Part model, mm, in its own coordinate system. Round coordinates to 2 decimals unless told otherwise and drop trailing zeros. Order: outer loops, then holes, each group sorted by start corner. A loop starts at its lowest first (then second) coordinate and runs counter-clockwise, first axis right, second up. Notation, with made-up numbers: (82.5, -24.75) - (104.5, -24.75) arc R29 ccw to (104.5, 1.25) - close; hole circle Ø9 at (25.25, 41.25). An arc over 180 degrees is marked (long way). Answer as a JSON object with one key per item and string values.
Autodesk Inventor part; units mm, degrees
ref_plane "YZ Plane" through (0, 0, 0) normal (1, 0, 0) x (0, 1, 0)
ref_plane "XZ Plane" through (0, 0, 0) normal (0, 1, 0) x (-1, 0, 0)
ref_plane "XY Plane" through (0, 0, 0) normal (0, 0, 1) x (1, 0, 0)
sketch "Sketch1" plane through (0, 0, 0) normal (0, 1, 0) x (-1, 0, 0)
  line L0 (0, 0) -> (28.63, 0)
  line L1 (28.63, 0) -> (28.63, -41.25) construction
  line L2 (28.63, -41.25) -> (0, -41.25)
  line L3 (0, -41.25) -> (0, 0)
  line L4 (28.63, 6.675) -> (31.43, 6.675)
  line L5 (31.43, 6.675) -> (31.43, 0)
  line L6 (31.43, -47.925) -> (28.63, -47.925)
  line L7 (28.63, -47.925) -> (28.63, -41.25)
  line L8 (31.43, -20.625) -> (28.63, -20.625) construction
  line L9 (38.98, 0) -> (31.43, 0)
  line L10 (31.43, 0) -> (31.43, -41.25) construction
  line L11 (31.43, -41.25) -> (35.18, -41.25)
  line L12 (38.98, -41.25) -> (38.98, -34.5) construction
  line L13 (31.43, -41.25) -> (35.18, -41.25) construction
  line L14 (38.98, 0) -> (38.98, -1) construction
  line L15 (38.98, -34.5) -> (35.18, -41.25)
  line L16 (38.98, -34.5) -> (38.98, -33)
  line L17 (35.18, -41.25) -> (38.98, -41.25) construction
  line L18 (38.98, 0) -> (38.98, -1) construction
  line L19 (38.98, -1) -> (39.98, -1)
  line L20 (39.98, -1) -> (39.98, -4)
  line L21 (39.98, -33) -> (38.98, -33)
  line L22 (38.98, -33) -> (38.98, -1) construction
  line L23 (38.98, -1) -> (38.98, -33) construction
  line L24 (38.98, -33) -> (38.98, -34.5) construction
  line L25 (38.98, -1) -> (38.98, 0)
  line L26 (38.98, -33) -> (38.98, -1) construction
  line L27 (31.43, 0) -> (31.43, -41.25) construction
  line L28 (31.43, -41.25) -> (31.43, -47.925)
  line L29 (28.63, -41.25) -> (28.63, 0) construction
  line L30 (28.63, 0) -> (28.63, 6.675)
  line L31 (28.63, 0) -> (31.43, 0) construction
  line L32 (31.43, -41.25) -> (28.63, -41.25) construction
  line L33 (39.98, -1) -> (39.98, -4) construction
  line L34 (39.98, -4) -> (41.28, -4)
  line L35 (41.28, -4) -> (41.28, -16.6)
  line L36 (41.28, -16.6) -> (39.98, -16.6)
  line L37 (39.98, -16.6) -> (39.98, -4) construction
  line L38 (39.98, -4) -> (39.98, -16.6) construction
  line L39 (39.98, -16.6) -> (39.98, -33)
  line L40 (41.68, -17) -> (41.68, -3.6)
  line L41 (41.68, -3.6) -> (40.38, -3.6)
  line L42 (40.38, -3.6) -> (40.38, -0.6)
  line L43 (40.38, -0.6) -> (39.38, -0.6)
  line L44 (39.38, -0.6) -> (39.38, 0.4)
  line L45 (39.38, 0.4) -> (31.83, 0.4)
  line L46 (31.83, 0.4) -> (31.83, 7.075)
  line L47 (31.83, 7.075) -> (28.23, 7.075)
  line L48 (28.23, 7.075) -> (28.23, 0.4)
  line L49 (28.23, 0.4) -> (-0.4, 0.4)
  line L50 (-0.4, 0.4) -> (-0.4, -41.65)
  line L51 (-0.4, -41.65) -> (28.23, -41.65)
  line L52 (28.23, -41.65) -> (28.23, -48.325)
  line L53 (28.23, -48.325) -> (31.83, -48.325)
  line L54 (31.83, -48.325) -> (31.83, -41.65)
  line L55 (31.83, -41.65) -> (35.4138, -41.65)
  line L56 (35.4138, -41.65) -> (39.38, -34.6049)
  line L57 (39.38, -34.6049) -> (39.38, -33.4)
  line L58 (39.38, -33.4) -> (40.38, -33.4)
  line L59 (40.38, -33.4) -> (40.38, -17)
  line L60 (40.38, -17) -> (41.68, -17)
  line L61 (0, -20.625) -> (39.98, -20.625) construction
  line L62 (44.99, 9.375) -> (-5.01, 9.375)
  line L63 (-5.01, 9.375) -> (-5.01, -50.625)
  line L64 (-5.01, -50.625) -> (44.99, -50.625)
  line L65 (44.99, -50.625) -> (44.99, 9.375)
  line L66 (19.99, 9.375) -> (19.99, -50.625) construction
  point P0 (30.03, 6.675)
  point P1 (19.99, -20.625)
  dimension "d0" = 28.63
  dimension "d1" = 41.25
  dimension "d2" = 2.8
  dimension "d3" = 54.6
  dimension "d4" = 7.55
  dimension "d5" = 41.25
  dimension "d6" = 3.75
  dimension "d7" = 34.5
  dimension "d8" = 1
  dimension "d9" = 32
  dimension "d10" = 1
  dimension "d11" = 6.675
  dimension "d12" = 3
  dimension "d13" = 1.3
  dimension "d14" = 12.6
  dimension "d15" = 0.4
  dimension "d16" = 50
  dimension "d17" = 60
extrude "Extrusion1" add sketch "Sketch1" along normal blind 5 contours L65 L64 L63 L62
sketch "Sketch2" plane through (0, 5, 0) normal (0, 1, 0) x (1, 0, 0)
  line L0 (-44.99, 50.625) -> (-44.99, -9.375)
  line L1 (5.01, 50.625) -> (-44.99, 50.625)
  line L2 (-44.99, -9.375) -> (-41.68, -9.375)
  line L3 (-41.68, -9.375) -> (-41.68, 50.625)
  line L4 (-41.68, 50.625) -> (-44.99, 50.625)
  line L5 (-44.99, 50.625) -> (-44.99, -9.375)
  point P0 (0, 0)
  dimension "d20" = 3.31
extrude "Extrusion2" cut sketch "Sketch2" against normal through all
sketch "Sketch3" plane through (0, 0, 0) normal (0, -1, 0) x (1, 0, 0)
  line L0 (5.01, 9.375) -> (5.01, -50.625)
  line L1 (-41.68, -17) -> (-41.68, -50.625)
  line L2 (5.01, 9.375) -> (-41.68, 9.375)
  line L3 (-41.68, 9.375) -> (-41.68, -50.625)
  line L4 (-41.68, -50.625) -> (5.01, -50.625)
  line L5 (5.01, -50.625) -> (5.01, 9.375)
  point P0 (0, 0)
extrude "Extrusion3" add sketch "Sketch3" along normal blind 4
sketch "Sketch4" plane through (-41.68, 5, 9.375) normal (0, 0, 1) x (1, 0, 0)
  line L0 (0, 0) -> (0, -9)
  line L1 (46.69, -9) -> (46.69, 0)
  line L2 (0, 0) -> (46.69, 0)
  line L3 (46.69, 0) -> (46.69, -9)
  line L4 (46.69, -9) -> (0, -9)
  line L5 (0, -9) -> (0, 0)
  point P0 (41.68, -5)
extrude "Extrusion4" add sketch "Sketch4" along normal blind 10
sketch "Sketch5" plane through (5.01, 5, -50.625) normal (0, 0, -1) x (-1, 0, 0)
  line L0 (0, 0) -> (46.69, 0)
  line L1 (46.69, 0) -> (46.69, -9)
  line L2 (0, 0) -> (46.69, 0)
  line L3 (46.69, 0) -> (46.69, -9)
  line L4 (46.69, -9) -> (0, -9)
  line L5 (0, -9) -> (0, 0)
  point P0 (5.01, -5)
extrude "Extrusion5" add sketch "Sketch5" along normal blind 10
sketch "Sketch6" plane through (0, -4, 0) normal (0, -1, 0) x (1, 0, 0)
  line L0 (-41.68, 19.375) -> (5.01, 19.375)
  line L1 (5.01, 19.375) -> (0.01, 19.375)
  line L2 (0.01, 14.375) -> (0.01, 10.375)
  line L3 (0.01, 10.375) -> (5.01, 10.375)
  line L4 (5.01, 10.375) -> (5.01, 19.375)
  line L5 (5.01, 19.375) -> (-3.99, 19.375)
  line L6 (-3.99, 19.375) -> (-3.99, 14.375)
  line L7 (-3.99, 14.375) -> (0.01, 14.375)
  line L8 (5.01, 14.375) -> (5.01, 19.375)
  point P0 (0, 0)
  dimension "d29" = 5
  dimension "d30" = 9
  dimension "d31" = 9
  dimension "d32" = 5
extrude "Extrusion6" add sketch "Sketch6" along normal blind 60
sketch "Sketch7" plane through (0, -4, 0) normal (0, -1, 0) x (1, 0, 0)
  line L0 (5.01, -60.625) -> (5.01, 19.375)
  line L1 (5.01, -60.625) -> (-3.99, -60.625)
  line L2 (-3.99, -60.625) -> (-3.99, -55.625)
  line L3 (-3.99, -55.625) -> (0.01, -55.625)
  line L4 (5.01, -55.625) -> (5.01, -60.625)
  line L5 (5.01, -60.625) -> (0.01, -60.625)
  line L6 (0.01, -55.625) -> (0.01, -51.625)
  line L7 (0.01, -51.625) -> (5.01, -51.625)
  line L8 (5.01, -51.625) -> (5.01, -60.625)
  line L9 (-41.68, -60.625) -> (-41.68, 19.375)
  line L10 (-41.68, -60.625) -> (-32.68, -60.625)
  line L11 (-32.68, -60.625) -> (-32.68, -55.625)
  line L12 (-32.68, -55.625) -> (-36.68, -55.625)
  line L13 (-41.68, -55.625) -> (-41.68, -60.625)
  line L14 (-41.68, -60.625) -> (-36.68, -60.625)
  line L15 (-36.68, -55.625) -> (-36.68, -51.625)
  line L16 (-36.68, -51.625) -> (-41.68, -51.625)
  line L17 (-41.68, -51.625) -> (-41.68, -60.625)
  line L18 (-41.68, 19.375) -> (-32.68, 19.375)
  line L19 (-32.68, 19.375) -> (-32.68, 14.375)
  line L20 (-32.68, 14.375) -> (-36.68, 14.375)
  line L21 (-41.68, 14.375) -> (-41.68, 19.375)
  line L22 (-41.68, 19.375) -> (-36.68, 19.375)
  line L23 (-36.68, 14.375) -> (-36.68, 10.375)
  line L24 (-36.68, 10.375) -> (-41.68, 10.375)
  line L25 (-41.68, 10.375) -> (-41.68, 19.375)
  point P0 (0, 0)
  dimension "d35" = 9
  dimension "d36" = 5
  dimension "d37" = 5
  dimension "d38" = 9
  dimension "d39" = 9
  dimension "d40" = 5
  dimension "d41" = 5
  dimension "d42" = 9
  dimension "d43" = 9
  dimension "d44" = 5
  dimension "d45" = 5
  dimension "d46" = 9
extrude "Extrusion7" add sketch "Sketch7" along normal blind 60
sketch "Sketch8" plane through (0, -64, 0) normal (0, -1, 0) x (1, 0, 0)
  line L0 (24.4558, -81.1334) -> (-117.6901, -81.1334)
  line L1 (-117.6901, -81.1334) -> (-117.6901, 38.2506)
  line L2 (-117.6901, 38.2506) -> (24.4558, 38.2506)
  line L3 (24.4558, 38.2506) -> (24.4558, -81.1334)
  point P0 (0, 0)
extrude "Extrusion8" add sketch "Sketch8" along normal blind 2.5
sketch "Sketch9" plane through (0, -64, 0) normal (0, 1, 0) x (1, 0, 0)
  line L0 (-36.68, -10.375) -> (-36.68, -14.375)
  line L1 (0.01, 51.625) -> (0.01, 55.625)
  line L2 (-36.68, -14.375) -> (0.01, -14.375)
  line L3 (0.01, -14.375) -> (0.01, 55.625)
  line L4 (0.01, 55.625) -> (-36.68, 55.625)
  line L5 (-36.68, 55.625) -> (-36.68, -14.375)
  line L6 (-3.99, -19.375) -> (-32.68, -19.375)
  line L7 (-41.68, -10.375) -> (-41.68, 51.625)
  line L8 (-3.99, 60.625) -> (5.01, 60.625)
  line L9 (-32.68, 60.625) -> (-3.99, 60.625)
  line L10 (5.01, 51.5309) -> (5.01, -10.375)
  point P0 (0, 0)
extrude "Extrusion9" cut sketch "Sketch9" against normal blind 2.5
sketch "Sketch10" plane through (0, -64, 0) normal (0, 1, 0) x (1, 0, 0)
  line L0 (0.01, -10.375) -> (5.01, -10.375)
  line L1 (5.01, 51.625) -> (0.01, 51.625)
  line L2 (0.01, -10.375) -> (5.01, -10.375)
  line L3 (5.01, -10.375) -> (5.01, 51.625)
  line L4 (5.01, 51.625) -> (0.01, 51.625)
  line L5 (0.01, 51.625) -> (0.01, -10.375)
  line L6 (-3.99, 55.625) -> (-3.99, 60.625)
  line L7 (-32.68, 60.625) -> (-32.68, 55.625)
  line L8 (-3.99, 60.625) -> (-32.68, 60.625)
  line L9 (-32.68, 60.625) -> (-32.68, 55.625)
  line L10 (-32.68, 55.625) -> (-3.99, 55.625)
  line L11 (-3.99, 55.625) -> (-3.99, 60.625)
  line L12 (-36.68, 55.625) -> (-36.68, -14.375)
  line L13 (-36.68, 51.625) -> (-41.6778, 51.625)
  line L14 (-41.6778, 51.625) -> (-41.6778, -10.375)
  line L15 (-41.6778, -10.375) -> (-36.68, -10.375)
  line L16 (-36.68, -10.375) -> (-36.68, 51.625)
  line L17 (-3.99, -14.375) -> (-32.68, -14.375)
  line L18 (-32.68, -14.375) -> (-3.99, -14.375)
  line L19 (-3.99, -14.375) -> (-3.99, -19.375)
  line L20 (-3.99, -19.375) -> (-32.68, -19.375)
  line L21 (-32.68, -19.375) -> (-32.68, -14.375)
  point P0 (0, 0)
extrude "Extrusion10" cut sketch "Sketch10" against normal blind 2.5
fillet "Fillet1" radius 2 5 edges at (-3.99, -65.25, -60.625) (0.01, -35.25, -55.625) (0.01, -35.25, -51.625) (-3.99, -35.25, -55.625) (5.01, -65.25, -51.625)
fillet "Fillet2" radius 2 10 edges at (5.01, -65.25, 10.375) (0.01, -35.25, 10.375) (0.01, -35.25, 14.375) (-3.99, -35.25, 14.375) (-3.99, -65.25, 19.375) (-32.68, -65.25, 19.375) (-32.68, -35.25, 14.375) (-36.68, -35.25, 14.375) (-36.68, -35.25, 10.375) (-41.6778, -65.25, 10.375)
fillet "Fillet3" radius 2 5 edges at (-36.68, -35.25, -51.625) (-36.68, -35.25, -55.625) (-32.68, -35.25, -55.625) (-32.68, -65.25, -60.625) (-41.6778, -65.25, -51.625)
fillet "Fillet4" radius 2 8 edges at (-41.68, -64, -56.125) (-37.18, -64, -60.625) (-41.68, -64, 14.875) (-37.18, -64, 19.375) (0.51, -64, 19.375) (5.01, -64, 14.875) (5.01, -64, -56.125) (0.51, -64, -60.625)
equation "\"d5\" = d1"
properties part number "OMG_20kg_servo_side_profile(0.4mm)"
Item 1: Drop flat-ended pins along their axis: P1, Ø5.5, axis at x = -41, y = -25.5, coming from the -Z side (3 decimals); P2, Ø5.5, axis at y = 1.5, z = -46, coming from the +X side; P3, Ø1.5, axis at y = -31, z = -60, coming from the -X side. Give the stop position or say it passes through.
Taken from the geometry:
{"P1": "z = -60.625", "P2": "x = 5.01", "P3": "x = -41.68"}
Item 2: Probe L1, parallel to X at y = -29.5, z = -54; L2, parallel to X at y = -41, z = -60; L3, parallel to Y at x = 16, z = -19. List the from-to ranges inside material, lowest first. Write a range as from..to.
Taken from the geometry:
{"L1": "-41.68..-36.64, -0.03..5.01", "L2": "-41.68..-32.68, -3.99..5.01", "L3": "-66.5..-64"}
Item 3: Cut at B-B (z = -13). Write the cut outline in (x, y), plus the area to 3 significant figures.
Taken from the geometry:
{"outline": "(-117.69, -66.5) - (-41.68, -66.5) - (-41.68, -64) - (-117.69, -64) - close; (-41.68, -4) - (5.01, -4) - (5.01, 5) - (0.4, 5) - (0.4, 0) - (-41.68, 0) - close; (5.01, -66.5) - (24.46, -66.5) - (24.46, -64) - (5.01, -64) - close", "area": "448 mm2"}
Item 4: Cut at C-C (y = -51). State how many separate pieces and enclosed holes the cut face has, plus the area to 3 significant figures.
Taken from the geometry:
{"separate pieces": "4", "enclosed holes": "0", "area": "257 mm2"}
Item 5: Cut at D-D (z = 29.5). Write the cut outline in (x, y), plus the area to 3 significant figures.
Taken from the geometry:
{"outline": "(-117.69, -66.5) - (24.46, -66.5) - (24.46, -64) - (-117.69, -64) - close", "area": "355 mm2"}
Item 6: Cut at A-A (x = -25). Write the cut outline in (y, z) (3 decimals).
Taken from the geometry:
{"outline": "(-66.5, -81.133) - (-64, -81.133) - (-64, -60.625) - (-66.5, -60.625) - close; (-66.5, 19.375) - (-64, 19.375) - (-64, 38.251) - (-66.5, 38.251) - close; (-4, -60.625) - (5, -60.625) - (5, -41.65) - (0, -41.65) - (0, 0.4) - (5, 0.4) - (5, 19.375) - (-4, 19.375) - close"}
Item 7: Two-plate mould, pull along Z, no slides. Class faces 1 (the flat face through (-31.83, 2, -45)), 2 (the flat face through (-3, -28, 19.375)), 3 (the flat face through (-28.23, 2, 4)), 4 (the flat face through (-34, -28, -60.625)): pulls with the +Z half, pulls with the -Z half, needs draft (parallel to the pull), parting line crosses it, or undercut.
Taken from the geometry:
{"face 1": "undercut", "face 2": "pulls with the +Z half", "face 3": "undercut", "face 4": "pulls with the -Z half"}
